from build123d import *

# Parameters (mm, degrees)
SKETCH1_R           = 4.6
SKETCH1_R_2         = 2.8
BOSS_EXTRUDE1_DEPTH = 7
BOSS_EXTRUDE2_START = 7
SKETCH1_3_W         = 14
SKETCH1_3_H         = 18
SKETCH1_3_R         = 4.6
SKETCH1_3_R_2       = 2.8
BOSS_EXTRUDE2_DEPTH = 5
SKETCH2_R           = 1.6
BOSS_EXTRUDE3_DEPTH = 6
FILLET1_R           = 2


with BuildPart() as part:
    # Sketch1 → Boss-Extrude1 (new body)
    with BuildSketch(Plane(origin=(0, 0, 0), x_dir=(1, 0, 0), z_dir=(0, 1, 0))):
        Circle(SKETCH1_R)
        Circle(SKETCH1_R_2, mode=Mode.SUBTRACT)
    extrude(amount=BOSS_EXTRUDE1_DEPTH)

    # Sketch1_3 → Boss-Extrude2 (add)
    with BuildSketch(Plane(origin=(0, 0, 0), x_dir=(1, 0, 0), z_dir=(0, 1, 0)).offset(BOSS_EXTRUDE2_START)):
        Rectangle(SKETCH1_3_W, SKETCH1_3_H)
        Circle(SKETCH1_3_R, mode=Mode.SUBTRACT)
        Circle(SKETCH1_3_R)
        Circle(SKETCH1_3_R_2, mode=Mode.SUBTRACT)
        Circle(SKETCH1_3_R_2)
    extrude(amount=BOSS_EXTRUDE2_DEPTH)

    # Sketch2 → Boss-Extrude3 (add)
    with BuildSketch(Plane(origin=(0, 12, 0), x_dir=(1, 0, 0), z_dir=(0, 1, 0))):
        with Locations((0, 3)):
            Circle(SKETCH2_R)
        with Locations((0, -3)):
            Circle(SKETCH2_R)
    extrude(amount=BOSS_EXTRUDE3_DEPTH)

    # Fillet1
    fillet1_edges = [part.edges().sort_by_distance(p)[0] for p in [
        (-7, 9.5, -9),
        (-7, 9.5, 9),
        (7, 9.5, 9),
        (7, 9.5, -9),
    ]]
    fillet(fillet1_edges, radius=FILLET1_R)


solid = part.part
CAD build for the part. Positions are in the model's coordinates, mm. A direction names the side the tool comes from. Round coordinates to 2 decimals unless told otherwise and drop trailing zeros. Loops run counter-clockwise (first coordinate to the right, second up) from the corner with the lowest first, then second, coordinate; pieces in that order, holes last.
(1) Wall check: line 1 along Z through (x, y) = (0, 4.5); line 2 along Y through (x, z) = (6, -3.25). Give the ranges that are in metal, low to high.
(2) Drop flat-ended pins along their axis: pin 1 (1.5 mm diameter, centred on x = -2.5, y = 5.5, fed in from +Z); pin 2 (4 mm diameter, centred on x = 2.5, y = 16, fed in from +Z). Give the stop position or say it passes through.
(3) Cut at D-D (x = -2). Give the cut face in (y, z).
(4) Two-plate mould, pull along Z, no slides. Class faces 4 (the cylindrical face through (-6.43, 9.54, 8.4)), 5 (the cylindrical face through (-3.65, 3.45, 2.8)), 6 (the flat face through (0, 18, -3)), 7 (the flat face through (0, 7, 0)): +Z half, -Z half, draft (parallel to the pull), parting line (faces both ways), or undercut.
(5) Cut at C-C (y = 3). Give the cut face in (x, z), plus the area to 3 significant figures.
(6) Which spindle directions (+Z, -Z, +X, -X, +Y, -Y) get a long thin tool onto all of the face, cutting with end or side? Do faces 1 (the cylindrical face through (-0.35, 14.96, 4.56)), 2 (the cylindrical face through (-2.8, 3.5, -0.1)), 3 (the flat face through (0, 9, -9)). Say none if no direction does.
(7) Cut at A-A (x = 0). Give the cut face in (y, z), plus the area to 3 significant figures.
(8) Cut at B-B (z = 0). Give the cut face in (x, y), plus the area to 3 significant figures.
Findings below:
1. line 1: z = -4.6 to -2.8, 2.8 to 4.6
1. line 2: y = 7 to 12
2. pin 1: stops at z = 4.25
2. pin 2: stops at z = 4.52
3. outline: (0, -4.14) - (7, -4.14) - (7, -9) - (12, -9) - (12, 9) - (7, 9) - (7, 4.14) - (0, 4.14) - (0, 1.96) - (7, 1.96) - (7, -1.96) - (0, -1.96) - close
4. face 4: +Z half
4. face 5: parting line
4. face 6: draft
4. face 7: undercut
5. outline: circle Ø9.2 at (0, 0); hole circle Ø5.6 at (0, 0)
5. area: 41.8 mm2
6. face 1: +Y
6. face 2: -Y
6. face 3: -Z, +X, -X, +Y, -Y
7. outline: (0, -4.6) - (7, -4.6) - (7, -9) - (12, -9) - (12, -4.6) - (18, -4.6) - (18, -1.4) - (12, -1.4) - (12, 1.4) - (18, 1.4) - (18, 4.6) - (12, 4.6) - (12, 9) - (7, 9) - (7, 4.6) - (0, 4.6) - (0, 2.8) - (7, 2.8) - (7, -2.8) - (0, -2.8) - close
7. area: 154 mm2
8. outline: (-7, 7) - (-4.6, 7) - (-4.6, 0) - (-2.8, 0) - (-2.8, 7) - (2.8, 7) - (2.8, 0) - (4.6, 0) - (4.6, 7) - (7, 7) - (7, 12) - (-7, 12) - close
8. area: 95.2 mm2
